Autodesk Inventor part; units mm, degrees
ref_plane "YZ Plane" through (0, 0, 0) normal (1, 0, 0) x (0, 1, 0)
ref_plane "XZ Plane" through (0, 0, 0) normal (0, 1, 0) x (-1, 0, 0)
ref_plane "XY Plane" through (0, 0, 0) normal (0, 0, 1) x (1, 0, 0)
sketch "Boceto1" plane through (0, 0, 0) normal (0, 1, 0) x (-1, 0, 0)
  line L0 (50, 100) -> (50, -100)
  line L1 (-50, 100) -> (50, -100) construction
  line L2 (50, 100) -> (-50, -100) construction
  line L3 (25, 100) -> (25, 97)
  line L4 (25, 97) -> (-25, 97)
  line L5 (-25, 97) -> (-25, 100)
  line L6 (-50, 100) -> (-25, 100)
  line L7 (25, 100) -> (50, 100)
  line L8 (25, -100) -> (25, -97)
  line L9 (25, -97) -> (-25, -97)
  line L10 (-25, -97) -> (-25, -100)
  line L11 (50, -100) -> (25, -100)
  line L12 (-25, -100) -> (-50, -100)
  line L13 (-50, -100) -> (-50, 100)
  point P0 (0, 0)
  dimension "d0" = 100
  dimension "d1" = 200
  dimension "d4" = 3
  dimension "d5" = 50
  dimension "d7" = 3
  dimension "d8" = 50
  dimension "d12" = 25
extrude "Extrusión1" add sketch "Boceto1" along normal blind 3
sketch "Boceto2" plane through (0, 3, 0) normal (0, 1, 0) x (1, 0, 0)
  line L0 (33, 12) -> (30, 12)
  line L1 (30, 12) -> (30, -38)
  line L2 (30, -38) -> (33, -38)
  line L3 (33, -38) -> (33, 12)
  line L4 (50, 100) -> (25, 100)
  line L5 (-50, 100) -> (-50, -100)
  point P0 (0, 0)
  dimension "d17" = 3
  dimension "d18" = 50
  dimension "d19" = 88
  dimension "d20" = 80
extrude "Extrusión2" cut sketch "Boceto2" against normal blind 3
sketch "Boceto3" plane through (0, 0, 0) normal (0, -1, 0) x (1, 0, 0)
  line L0 (-40, -1.5) -> (-10, -1.5)
  line L1 (-10, -1.5) -> (-10, 1.5)
  line L2 (-10, 1.5) -> (-40, 1.5)
  line L3 (-40, 1.5) -> (-40, -1.5)
  line L4 (-50, -100) -> (-25, -100)
  line L5 (30, -12) -> (30, 38)
  point P0 (0, 0)
  dimension "d23" = 30
  dimension "d24" = 3
  dimension "d25" = 98.5
  dimension "d26" = 40
extrude "Extrusión3" cut sketch "Boceto3" against normal blind 3
sketch "Boceto4" plane through (0, 0, 0) normal (0, -1, 0) x (1, 0, 0)
  line L0 (23.5, 16.5) -> (26.5, 16.5)
  line L1 (26.5, 16.5) -> (26.5, 36.5)
  line L2 (26.5, 36.5) -> (23.5, 36.5)
  line L3 (23.5, 36.5) -> (23.5, 16.5)
  line L4 (-40, 1.5) -> (-10, 1.5)
  line L5 (30, -12) -> (30, 38)
  point P0 (0, 0)
  dimension "d29" = 3
  dimension "d30" = 20
  dimension "d31" = 15
  dimension "d32" = 3.5
extrude "Extrusión4" cut sketch "Boceto4" against normal blind 3
properties part number "Piso"
Input: part model. Units: mm. Frame: model coordinates. Round coordinates to 2 decimals unless told otherwise and drop trailing zeros. Order: outer loops, then holes, each group sorted by start corner. A loop starts at its lowest first (then second) coordinate and runs counter-clockwise, first axis right, second up. Notation, with made-up numbers: (69, -4.75) - (114, -4.75) arc R28 cw to (114, 30.25) - close; hole circle Ø10 at (-11, -16). An arc over 180 degrees is marked (long way). Answer as a JSON object with one key per item and string values. Group by question number.
(1) Material intervals for probe 1 along Z at (x, y) = (-26.5, 2.6); probe 2 along Z at (x, y) = (-18.5, 2.15); probe 3 along X at (y, z) = (1.4, 9.5), sorted ascending. Write a range as from..to.
(2) Pin query (flat end, axial travel): P1, Ø0.9, axis at x = 2.5, y = 1, coming from the -Z side; P2, Ø1.5, axis at x = -24, y = 1, coming from the +Z side. Return the tip coordinate at first contact, or that it passes through.
(3) Cut plane A-A (x = -16.5). Return loops of the section in (y, z), then the cut area to 3 significant figures.
(4) Cut plane D-D (y = 2.55). Return loops of the section in (x, z), then the cut area to 3 significant figures.
(5) Cut plane B-B (z = 33). Return loops of the section in (x, y), then the cut area to 3 significant figures.
(6) Cut plane C-C (z = -6). Return loops of the section in (x, y).
Here are the results:
{
 "1": {"probe 1": "z = -100..-1.5, 1.5..100", "probe 2": "z = -97..-1.5, 1.5..97", "probe 3": "x = -50..30, 33..50"},
 "2": {"P1": "stops at z = -97", "P2": "stops at z = 97"},
 "3": {"outline": "(0, -97) - (3, -97) - (3, -1.5) - (0, -1.5) - close; (0, 1.5) - (3, 1.5) - (3, 97) - (0, 97) - close", "area": "573 mm^2"},
 "4": {"outline": "(-50, -100) - (-25, -100) - (-25, -97) - (25, -97) - (25, -100) - (50, -100) - (50, 100) - (25, 100) - (25, 97) - (-25, 97) - (-25, 100) - (-50, 100) - close; hole (-40, -1.5) - (-10, -1.5) - (-10, 1.5) - (-40, 1.5) - close; hole (23.5, 16.5) - (26.5, 16.5) - (26.5, 36.5) - (23.5, 36.5) - close; hole (30, -12) - (33, -12) - (33, 38) - (30, 38) - close", "area": "19,400 mm^2"},
 "5": {"outline": "(-50, 0) - (23.5, 0) - (23.5, 3) - (-50, 3) - close; (26.5, 0) - (30, 0) - (30, 3) - (26.5, 3) - close; (33, 0) - (50, 0) - (50, 3) - (33, 3) - close", "area": "282 mm^2"},
 "6": {"outline": "(-50, 0) - (30, 0) - (30, 3) - (-50, 3) - close; (33, 0) - (50, 0) - (50, 3) - (33, 3) - close"}
}
